```python
from build123d import *

# Parameters (mm, degrees)
F2_R     = 46
F0_R     = 31.5
F4_T     = -2.54
F6_DEPTH = 68.58
F7_W     = 43.7282323837
F7_H     = 56.1075247824
F8_DEPTH = 66.04
F9_R     = 5.08
F10_R    = 2.0974699773


with BuildPart() as f3:
    # F2 (on offset) → F3 section 0
    with BuildSketch(Plane.XZ.offset(-190)):
        Circle(F2_R)
    # F0 (on Front) → F3 section 1
    with BuildSketch(Plane.XZ):
        Circle(F0_R)
    loft()

    # F4
    f4_openings = [f3.faces().sort_by_distance(p)[0] for p in [
        (0, 0, 0),
        (0, 190, 0),
    ]]
    offset(amount=F4_T, openings=f4_openings, kind=Kind.INTERSECTION)

    # F5 (on Top) → F6 (cut)
    with BuildSketch(Plane.XY):
        Polygon((-50.4529035675, 192.8699612617), (-43.8499934971, 145.5444693565), (0, 192.8699612617), align=None)
        Polygon((49.8117071029, 192.8699612617), (0, 192.8699612617), (44.228361635, 145.5444693565), align=None)
    extrude(amount=F6_DEPTH, mode=Mode.SUBTRACT)

    # F7 (on Right) → F8 (cut, symmetric)
    with BuildSketch(Plane.YZ):
        with Locations((168.6937212944, -28.0537623912)):
            Rectangle(F7_W, F7_H)
    extrude(amount=F8_DEPTH, both=True, mode=Mode.SUBTRACT)

    # F9
    f9_edges = [f3.edges().sort_by_distance(p)[0] for p in [
        (-2.659197, 190, 44.647121),
        (2.682142, 190, 44.645748),
    ]]
    fillet(f9_edges, radius=F9_R)

    # F10
    f10_edges = [f3.edges().sort_by_distance(p)[0] for p in [
        (-31.5, 0, 0),
    ]]
    fillet(f10_edges, radius=F10_R)


solid = f3.part
```
For this review, take the finished solid that the model builds, in its own axes (mm). Round coordinates to 2 decimals unless told otherwise and drop trailing zeros. Write each loop counter-clockwise with the first axis right and the second up, starting at its lowest first coordinate (ties: lowest second). Pieces come first, ordered by that corner, then holes.
1) For line 1 along X through (y, z) = (40, -16.5); line 2 along X through (y, z) = (79.5, 13); line 3 along Z through (x, y) = (-19, 26.5), list the stretches that pass through material, from the lowest coordinate up.
Answer below:
line 1: x = -30.36 to -27.42, 27.42 to 30.36
line 2: x = -35.25 to -32.52, 32.52 to 35.25
line 3: z = -27.62 to -24.46, 24.46 to 27.62
2) Take a section at B-B on y = 61.5. Give the boundary of the cut face in (x, z).
Answer below:
outline: circle Ø72.39 at (0, 0); hole circle Ø67.29 at (0, 0)
3) Insertion check: pin 1 Ø6 at (y, z) = (149, -7) entering from -X; pin 2 Ø2 at (x, y) = (41, 149) entering from -Z; pin 3 Ø1 at (y, z) = (145, 22.5) entering from -X. Each pin has a flat end and moves straight along its axis. Give the tip position at first contact, or say it passes through.
Answer below:
pin 1: stops at x = -42.42
pin 2: stops at z = 0
pin 3: stops at x = -36.44
4) Take a section at A-A on y = 19. Give the boundary of the cut face in (x, z), then the cut area to 3 significant figures.
Answer below:
outline: circle Ø65.9 at (0, 0); hole circle Ø60.81 at (0, 0)
area: 507 mm2
5) Mouldability with a two-part tool opening along X and no side actions: class faces 1 (the face through (30.506, 160.227, 29.504)), 2 (the face through (-4.5, 72.6, 34.2)), 3 (the face through (0.2, 146.83, -40.4)), 4 (the face through (-29.233, 161.32, 29.505)) as +X half, -X half, draft (parallel to the pull), parting line (faces both ways), or undercut.
Answer below:
face 1: +X half
face 2: undercut
face 3: draft
face 4: -X half
